Could you check a few things on this model? Use its own coordinates, in mm. A direction names the side the tool comes from. Round coordinates to 2 decimals unless told otherwise and drop trailing zeros. Loops run counter-clockwise (first coordinate to the right, second up) from the corner with the lowest first, then second, coordinate; pieces in that order, holes last. Notation, with made-up numbers: M -15,-27.75 L 33,-27.75 A26 ccw 33,-1.75 Z; hole C -18.5,-9.5 d2. An arc over 180 degrees is marked long. Answer in a Markdown table with one row per item.
```python
from build123d import *

# Parameters (mm, degrees)
SKETCH1_W           = 50.8
SKETCH1_H           = 127
BOSS_EXTRUDE1_DEPTH = 2.54
SKETCH2_R           = 15.875
BOSS_EXTRUDE2_DEPTH = 57.15
SKETCH3_W           = 50.8
SKETCH3_H           = 6.35
BOSS_EXTRUDE3_DEPTH = 50.8
BOSS_EXTRUDE4_DEPTH = 50.8


with BuildPart() as part:
    # Sketch1 → Boss-Extrude1 (new body)
    with BuildSketch(Plane.XY):
        Rectangle(SKETCH1_W, SKETCH1_H)
    extrude(amount=BOSS_EXTRUDE1_DEPTH)

    # Sketch2 → Boss-Extrude2 (add)
    with BuildSketch(Plane.XY.offset(2.54)):
        with Locations((0, 22.465516187)):
            Circle(SKETCH2_R)
        with Locations((0, -28.334483813)):
            Circle(SKETCH2_R)
    extrude(amount=BOSS_EXTRUDE2_DEPTH)

    # Sketch3 → Boss-Extrude3 (add)
    with BuildSketch(Plane(origin=(0, 0, 0), x_dir=(-1, 0, 0), z_dir=(0, 0, -1))):
        with Locations((0, -60.325)):
            Rectangle(SKETCH3_W, SKETCH3_H)
    extrude(amount=BOSS_EXTRUDE3_DEPTH)

    # Sketch4 → Boss-Extrude4 (add)
    with BuildSketch(Plane(origin=(25.4, 0, 0), x_dir=(0, 0, -1), z_dir=(1, 0, 0))):
        Polygon((44.45, -63.5), (60.482117808, -47.467882192), (54.66777369, -47.467882192), (38.635655882, -63.5), align=None)
    extrude(amount=-BOSS_EXTRUDE4_DEPTH)


solid = part.part
```
1) I want a section at D-D, the plane y = -3. Please give me the cut outline in (x, z).
Computed:
| item | result |
|---|---|
| outline | M -25.4,0 L 25.4,0 L 25.4,2.54 L -25.4,2.54 Z |
2) Which directions (+Z, -Z, +X, -X, +Y, -Y) give clear straight access to the entire face, cutting with the end or side of a thin tool? Please do faces 4 (the face through (0, -28, 59.69)), 5 (the face through (0, -47.468, -58)), 6 (the face through (-3.441, -43.832, 30.715)), 7 (the face through (0, -60, -50.8)), 8 (the face through (0, -57.15, -22)).
Computed:
| item | result |
|---|---|
| face 4 | +Z, +X, -X, +Y, -Y |
| face 5 | -Z, +X, -X, +Y |
| face 6 | +Z |
| face 7 | -Z, +X, -X, -Y |
| face 8 | +X, -X, +Y |
3) I need wall thicknesses on line 1 (Z direction, x = -5.5, y = 33); line 2 (Y direction, x = -0.5, z = 16); line 3 (Y direction, x = -18.5, z = -22). Which ranges of each line are inside material? Lowest first, please.
Computed:
| item | result |
|---|---|
| line 1 | z = 0 to 59.69 |
| line 2 | y = -44.2 to -12.47, 6.6 to 38.33 |
| line 3 | y = -63.5 to -57.15 |
4) If we mould it in two halves opening along Y, with no side actions, what happens to faces 1 (the face through (0, 1, 2.54)), 2 (the face through (0, -63.5, -24)), 3 (the face through (0, 23, 59.69))? For each: released by +Y, released by -Y, zero draft, split by the parting line, or undercut.
Computed:
| item | result |
|---|---|
| face 1 | undercut |
| face 2 | released by -Y |
| face 3 | zero draft |
5) Will these pins go through, and if not, where does the flat tip stop? P1, Ø3, axis at x = 14.5, y = 27.5, coming from the -Z side; P2, Ø5, axis at x = -8, z = 47.5, coming from the -Y side; P3, Ø7, axis at x = 5, y = -59, coming from the -Z side.
Computed:
| item | result |
|---|---|
| P1 | stops at z = 0 |
| P2 | stops at y = -43.23 |
| P3 | stops at z = -52.45 |
6) I want a section at B-B, the plane x = 0. Please give me the cut outline in (y, z), plus the area to 3 significant figures.
Computed:
| item | result |
|---|---|
| outline | M -63.5,-50.8 L -57.15,-50.8 L -47.47,-60.48 L -47.47,-54.67 L -57.15,-44.99 L -57.15,0 L 63.5,0 L 63.5,2.54 L 38.34,2.54 L 38.34,59.69 L 6.59,59.69 L 6.59,2.54 L -12.46,2.54 L -12.46,59.69 L -44.21,59.69 L -44.21,2.54 L -63.5,2.54 Z |
| area | 4,330 mm² |
7) I want a section at A-A, the plane y = -51. Please give me the cut outline in (x, z), plus the area to 3 significant figures.
Computed:
| item | result |
|---|---|
| outline | M -25.4,-56.95 L 25.4,-56.95 L 25.4,-51.14 L -25.4,-51.14 Z; M -25.4,0 L 25.4,0 L 25.4,2.54 L -25.4,2.54 Z |
| area | 424 mm² |
8) I want a section at C-C, the plane z = -15.5. Please give me the cut outline in (x, y), plus the area to 3 significant figures.
Computed:
| item | result |
|---|---|
| outline | M -25.4,-63.5 L 25.4,-63.5 L 25.4,-57.15 L -25.4,-57.15 Z |
| area | 323 mm² |
